Work out the finished part from the listing and answer in its coordinate system (mm). A direction names the side the tool comes from. Coordinates: 2 decimals unless noted, no trailing zeros. Loops run counter-clockwise (first coordinate to the right, second up) from the corner with the lowest first, then second, coordinate; pieces in that order, holes last. Notation, with made-up numbers: (-6, 5.25) -> (52, 5.25) arc R24 ccw to (52, 39.25) -> close; hole circle Ø3 at (-5, 85). An arc over 180 degrees is marked (long way). Use a Markdown table: item, result.
Autodesk Inventor part; units mm, degrees
ref_plane "Work Plane1" through (5.08, 0, 0) normal (1, 0, 0) x (0, 1, 0)
ref_plane "Work Plane2" through (3.81, 0, 0) normal (1, 0, 0) x (0, 1, 0)
ref_plane "XZ Plane" through (0, 0, 0) normal (0, 1, 0) x (-1, 0, 0)
ref_plane "Work Plane1" through (5.08, 0, 0) normal (1, 0, 0) x (0, 1, 0)
sketch "Sketch2" plane through (5.08, 0, 0) normal (1, 0, 0) x (0, 1, 0)
  circle A0 centre (0, 0) radius 3.81
  dimension "d2" = 7.62
extrude "Extrusion1" add sketch "Sketch2" along normal blind 5.715
ref_plane "Work Plane2" through (3.81, 0, 0) normal (1, 0, 0) x (0, 1, 0)
sketch "Sketch3" plane through (3.81, 0, 0) normal (1, 0, 0) x (0, 1, 0)
  circle A0 centre (0, 0) radius 4.445
  dimension "d6" = 8.89
loft "Loft1" add profiles "Sketch3" section 2 edges at (5.08, -3.81, 0)
extrude "Extrusion2" add sketch "Sketch3" against normal blind 4.445
mirror "Mirror1" about plane through (10.795, 0, 0) normal (1, 0, 0) of "Extrusion1", "Loft1", "Extrusion2"
shell "Shell1" thickness 1.27 removed faces 1 at (22.225, 1.6691, 0.6886)
fillet "Fillet1" radius 3.175 6 edges at (3.81, -4.445, 0) (5.08, -3.81, 0) (16.51, -3.81, 0) (17.78, -4.445, 0) (4.7802, -2.54, 0) (16.8098, -2.54, 0)
chamfer "Chamfer1" distance 0.254 angle 45 2 edges at (-0.635, -4.445, 0) (22.225, -4.445, 0)
properties part number "Axle-Connector"
Q1. Given pin 1 Ø1.5 at (x, z) = (7, 3) entering from +Y; pin 2 Ø5 at (y, z) = (-0.5, 0) entering from +X; pin 3 Ø3 at (x, z) = (11, -1) entering from -Y, each flat-ended and moving along its own axis, determine where each tip first touches the part or whether it passes through.
Solved:
| item | result |
|---|---|
| pin 1 | y = 3.07 |
| pin 2 | x = 17.73 |
| pin 3 | y = -3.81 |
Q2. Consider line 1 (Y direction, x = 20.2, z = 0) (3 decimals); line 2 (Z direction, x = 10.25, y = 0). Determine where each line is inside the solid, lowest interval first. Write a range as [from, to].
Solved:
| item | result |
|---|---|
| line 1 | [-4.445, -3.175], [3.175, 4.445] |
| line 2 | [-3.81, -2.54], [2.54, 3.81] |
Q3. Determine the mould class of faces 4 (the flat face through (22.225, -2, 3)), 5 (the cylindrical face through (10.72, -0.33, -2.52)), 6 (the cylindrical face through (20.226, 2.051, 3.943)) for opening direction Y: pulls with the +Y half, pulls with the -Y half, needs draft (parallel to the pull), parting line crosses it, or undercut.
Solved:
| item | result |
|---|---|
| face 4 | needs draft |
| face 5 | undercut |
| face 6 | parting line crosses it |
Q4. For faces 1 (the cylindrical face through (2.09, -0.69, -3.1)), 2 (the flat face through (-0.635, 0, 0)), 3 (the cylindrical face through (20.12, -0.69, 3.1)), determine the directions among +Z, -Z, +X, -X, +Y, -Y from which every point of the face is accessible in a straight line to the end or side of a thin tool.
Solved:
| item | result |
|---|---|
| face 1 | none |
| face 2 | +Z, -Z, -X, +Y, -Y |
| face 3 | +X |
Q5. Section A-A on x = 10.5 is taken. Determine the outline of the cut face in (y, z).
Solved:
| item | result |
|---|---|
| outline | circle Ø7.62 at (0, 0); hole circle Ø5.08 at (0, 0) |
